The model under review builds one solid part; all positions refer to its coordinate system, in mm. Round coordinates to 2 decimals unless told otherwise and drop trailing zeros. Write each loop counter-clockwise with the first axis right and the second up, starting at its lowest first coordinate (ties: lowest second). Pieces come first, ordered by that corner, then holes. Notation, with made-up numbers: (-2, 39) -> (39, 39) arc R16 cw to (39, 70) -> close; hole circle Ø10 at (79.25, 8.5). An arc over 180 degrees is marked (long way). Return JSON: item names as keys, results as strings. Group by question number.
1. Take a section at A-A, the plane z = 2.75. Give the number of separate pieces and of enclosed holes in the cut face, then the cut area to 3 significant figures.
2. For line 1 along Y through (x, z) = (-13, 5); line 2 along X through (y, z) = (47.5, 5.5); line 3 along Y through (x, z) = (-27, 4), list the stretches that pass through material, from the lowest coordinate up. Write a range as from..to.
3. Take a section at B-B, the plane x = -6. Write out the cut boundary in (y, z), then the cut area to 3 significant figures.
from build123d import *

# Parameters (mm, degrees)
SKETCH1_W           = 76.2
SKETCH1_H           = 139.7
BOSS_EXTRUDE1_DEPTH = 6.35
SKETCH2_R           = 2.54
CUT_EXTRUDE1_DEPTH  = 15.24
SKETCH3_R           = 2.54
CUT_EXTRUDE2_DEPTH  = 15.24
SKETCH4_R           = 2.54
CUT_EXTRUDE3_DEPTH  = 7.62
CUT_EXTRUDE4_DEPTH  = 7.62


with BuildPart() as part:
    # Sketch1 → Boss-Extrude1 (new body)
    with BuildSketch(Plane.XY):
        with Locations((-13.133014553, 21.815443873)):
            Rectangle(SKETCH1_W, SKETCH1_H)
    extrude(amount=BOSS_EXTRUDE1_DEPTH)

    # Sketch2 → Cut-Extrude1 (cut)
    with BuildSketch(Plane(origin=(0, 0, 0), x_dir=(-1, 0, 0), z_dir=(0, 0, -1))):
        with Locations((45.518014553, 85.315443873)):
            Circle(SKETCH2_R)
        with Locations((45.518014553, 72.615443873)):
            Circle(SKETCH2_R)
        with Locations((45.518014553, -28.984556127)):
            Circle(SKETCH2_R)
        with Locations((45.518014553, -41.684556127)):
            Circle(SKETCH2_R)
        with Locations((-19.251985447, -41.684556127)):
            Circle(SKETCH2_R)
        with Locations((-19.251985447, -28.984556127)):
            Circle(SKETCH2_R)
        with Locations((-19.251985447, 85.315443873)):
            Circle(SKETCH2_R)
        with Locations((-19.251985447, 72.615443873)):
            Circle(SKETCH2_R)
    extrude(amount=-CUT_EXTRUDE1_DEPTH, mode=Mode.SUBTRACT)

    # Sketch3 → Cut-Extrude2 (cut)
    with BuildSketch(Plane.XY.offset(6.35)):
        with Locations((-19.483014553, 38.325443873)):
            Circle(SKETCH3_R)
        with Locations((-6.783014553, 38.325443873)):
            Circle(SKETCH3_R)
        with Locations((-19.483014553, 73.885443873)):
            Circle(SKETCH3_R)
        with Locations((-6.783014553, 73.885443873)):
            Circle(SKETCH3_R)
    extrude(amount=-CUT_EXTRUDE2_DEPTH, mode=Mode.SUBTRACT)

    # Sketch4 → Cut-Extrude3 (cut)
    with BuildSketch(Plane.XY.offset(6.35)):
        with Locations((-45.899014553, 49.755443873)):
            Circle(SKETCH4_R)
        with Locations((-45.899014553, -6.124556127)):
            Circle(SKETCH4_R)
        with Locations((19.632985447, -6.124556127)):
            Circle(SKETCH4_R)
        with Locations((19.632985447, 49.755443873)):
            Circle(SKETCH4_R)
    extrude(amount=-CUT_EXTRUDE3_DEPTH, mode=Mode.SUBTRACT)

    # Sketch5 → Cut-Extrude4 (cut)
    with BuildSketch(Plane(origin=(0, 0, 0), x_dir=(-1, 0, 0), z_dir=(0, 0, -1))):
        with BuildLine():
            Line((0.433014553, 25.625443873), (25.833014553, 25.625443873))
            ThreePointArc((25.833014553, 25.625443873), (28.373014553, 23.085443873), (25.833014553, 20.545443873))
            Line((25.833014553, 20.545443873), (0.433014553, 20.545443873))
            ThreePointArc((0.433014553, 20.545443873), (-2.106985447, 23.085443873), (0.433014553, 25.625443873))
        make_face()
        with BuildLine():
            Line((0.433014553, -31.524556127), (25.833014553, -31.524556127))
            ThreePointArc((25.833014553, -31.524556127), (28.373014553, -34.064556127), (25.833014553, -36.604556127))
            Line((25.833014553, -36.604556127), (0.433014553, -36.604556127))
            ThreePointArc((0.433014553, -36.604556127), (-2.106985447, -34.064556127), (0.433014553, -31.524556127))
        make_face()
    extrude(amount=-CUT_EXTRUDE4_DEPTH, mode=Mode.SUBTRACT)


solid = part.part
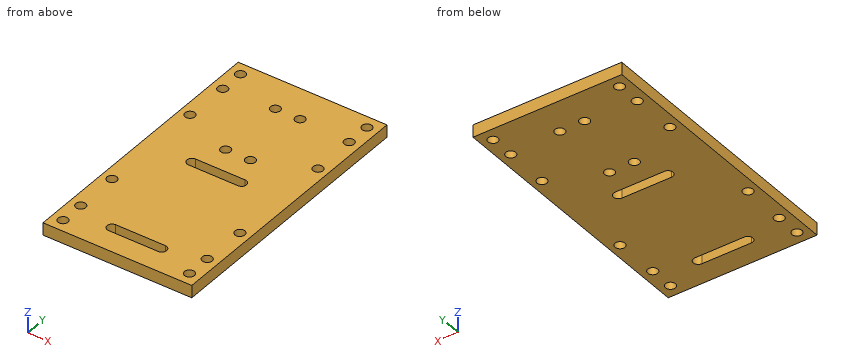
Output:
{
 "1": {"separate pieces": "1", "enclosed holes": "18", "area": "10,000 mm^2"},
 "2": {"line 1": "y = -48.03..-36.6, -31.52..20.55, 25.63..91.67", "line 2": "x = -51.23..-47.07, -44.73..18.46, 20.8..24.97", "line 3": "y = -48.03..-36.32, -31.81..20.83, 25.34..91.67"},
 "3": {"outline": "(-48.03, 0) -> (-36.6, 0) -> (-36.6, 6.35) -> (-48.03, 6.35) -> close; (-31.52, 0) -> (20.55, 0) -> (20.55, 6.35) -> (-31.52, 6.35) -> close; (25.63, 0) -> (35.91, 0) -> (35.91, 6.35) -> (25.63, 6.35) -> close; (40.74, 0) -> (71.47, 0) -> (71.47, 6.35) -> (40.74, 6.35) -> close; (76.3, 0) -> (91.67, 0) -> (91.67, 6.35) -> (76.3, 6.35) -> close", "area": "761 mm^2"}
}
